The model under review builds one solid part; all positions refer to its coordinate system, in mm. A direction names the side the tool comes from. Round coordinates to 2 decimals unless told otherwise and drop trailing zeros. Write each loop counter-clockwise with the first axis right and the second up, starting at its lowest first coordinate (ties: lowest second). Pieces come first, ordered by that corner, then holes. Notation, with made-up numbers: M -2,53 L 19,53 A15 ccw 19,69 Z; hole C 75.25,56.5 d10. An arc over 180 degrees is marked long. One line per item, written item: value. Start each with the question number.
1) Take a section at D-D, the plane x = 79. Write out the cut boundary in (y, z).
2) Mouldability with a two-part tool opening along X and no side actions: class faces 3 (the face through (60.81, 6.44, 7.5)), 4 (the face through (0, 0, 7)) as +X half, -X half, draft (parallel to the pull), parting line (faces both ways), or undercut.
3) Take a section at B-B, the plane y = 5.25. Write out the cut boundary in (x, z) (3 decimals).
4) Take a section at C-C, the plane z = -51.5. Write out the cut boundary in (x, y), and give its area (3 significant figures).
5) Take a section at A-A, the plane x = 0. Write out the cut boundary in (y, z) (3 decimals).
6) Wall thickness on probe 1 along Z at (x, y) = (38, 3.5); probe 2 along X at (y, z) = (10, 66); probe 3 along X at (y, z) = (4.75, -38): over which ranges is each line inside the solid? List them lowest first.
7) For P1, Ø6, axis at x = 19.5, y = 9.5, coming from the -Z side; P2, Ø2, axis at y = 4.5, z = -45.5, coming from the +X side; P3, Ø1.5, axis at x = 16, y = 4, coming from the +Z side, all flat-tipped, find the tip position at first contact; note any pin that passes through.
8) Tool access review of faces 1 (the face through (0, 12.7, 7)), 2 (the face through (36.3, 6.4, -48.2)): name each direction out of +Z, -Z, +X, -X, +Y, -Y from which nothing blocks a thin tool from reaching the whole face with its end or side.
from build123d import *

# Parameters (mm, degrees)
SKETCH1_R           = 98.425
BOSS_EXTRUDE1_DEPTH = 12.7
CUT_EXTRUDE1_DEPTH  = 13.7


with BuildPart() as part:
    # Sketch1 → Boss-Extrude1 (new body)
    with BuildSketch(Plane(origin=(0, 0, 0), x_dir=(1, 0, 0), z_dir=(0, 1, 0))):
        Circle(SKETCH1_R)
    extrude(amount=BOSS_EXTRUDE1_DEPTH)

    # Sketch2 → Cut-Extrude1 (cut, through all)
    with BuildSketch(Plane(origin=(0, 12.7, 0), x_dir=(1, 0, 0), z_dir=(0, 1, 0))):
        with BuildLine():
            Line((21.383254088, 20.544146731), (61.581662722, 68.450744637))
            ThreePointArc((61.581662722, 68.450744637), (86.522198059, 31.491504697), (91.173581053, -12.852382775))
            Line((91.173581053, -12.852382775), (29.586045941, -1.992838659))
            ThreePointArc((29.586045941, -1.992838659), (27.864786272, 10.141952787), (21.383254088, 20.544146731))
        make_face()
        with BuildLine():
            Line((16.518871875, 24.625848052), (56.717280509, 72.532445958))
            ThreePointArc((56.717280509, 72.532445958), (15.988655959, 90.676173859), (-28.489252402, 87.556656643))
            Line((-28.489252402, 87.556656643), (-7.100125924, 28.790514622))
            ThreePointArc((-7.100125924, 28.790514622), (5.149204378, 29.202589176), (16.518871875, 24.625848052))
        make_face()
        with BuildLine():
            Line((-13.067174066, 26.618686712), (-34.456300544, 85.384828733))
            ThreePointArc((-34.456300544, 85.384828733), (-70.5335421, 59.184669162), (-90.070915125, 19.105912006))
            Line((-90.070915125, 19.105912006), (-28.483380012, 8.246367891))
            ThreePointArc((-28.483380012, 8.246367891), (-22.715581894, 19.060636389), (-13.067174066, 26.618686712))
        make_face()
        with BuildLine():
            Line((-29.586045941, 1.992838659), (-91.173581053, 12.852382775))
            ThreePointArc((-91.173581053, 12.852382775), (-86.522198059, -31.491504697), (-61.581662722, -68.450744637))
            Line((-61.581662722, -68.450744637), (-21.383254088, -20.544146731))
            ThreePointArc((-21.383254088, -20.544146731), (-27.864786272, -10.141952787), (-29.586045941, 1.992838659))
        make_face()
        with BuildLine():
            Line((-16.518871875, -24.625848052), (-56.717280509, -72.532445958))
            ThreePointArc((-56.717280509, -72.532445958), (-15.988655959, -90.676173859), (28.489252402, -87.556656643))
            Line((28.489252402, -87.556656643), (7.100125924, -28.790514622))
            ThreePointArc((7.100125924, -28.790514622), (-5.149204378, -29.202589176), (-16.518871875, -24.625848052))
        make_face()
        with BuildLine():
            Line((13.067174066, -26.618686712), (34.456300544, -85.384828733))
            ThreePointArc((34.456300544, -85.384828733), (70.5335421, -59.184669162), (90.070915125, -19.105912006))
            Line((90.070915125, -19.105912006), (28.483380012, -8.246367891))
            ThreePointArc((28.483380012, -8.246367891), (22.715581894, -19.060636389), (13.067174066, -26.618686712))
        make_face()
    extrude(amount=-CUT_EXTRUDE1_DEPTH, mode=Mode.SUBTRACT)


solid = part.part
Checked values:
1. outline: M 0,-58.71 L 12.7,-58.71 L 12.7,-47.29 L 0,-47.29 Z; M 0,10.71 L 12.7,10.71 L 12.7,17.15 L 0,17.15 Z; M 0,47.29 L 12.7,47.29 L 12.7,58.71 L 0,58.71 Z
2. face 3: undercut
2. face 4: draft
3. outline: C 0,0 d196.85; hole M -91.174,-12.852 L -29.586,-1.993 A29.653 cw -21.383,20.544 L -61.582,68.451 A92.075 ccw Z; hole M -90.071,-19.106 A92.075 ccw -34.456,-85.385 L -13.067,-26.619 A29.653 cw -28.483,-8.246 Z; hole M -56.717,72.532 L -16.519,24.626 A29.653 cw 7.1,28.791 L 28.489,87.557 A92.075 ccw Z; hole M -28.489,-87.557 A92.075 ccw 56.717,-72.532 L 16.519,-24.626 A29.653 cw -7.1,-28.791 Z; hole M 13.067,26.619 A29.653 cw 28.483,8.246 L 90.071,19.106 A92.075 ccw 34.456,85.385 Z; hole M 21.383,-20.544 L 61.582,-68.451 A92.075 ccw 91.174,12.852 L 29.586,1.993 A29.653 cw Z
4. outline: M -83.88,0 L -76.33,0 L -76.33,12.7 L -83.88,12.7 Z; M -22.12,0 L -15.37,0 L -15.37,12.7 L -22.12,12.7 Z; M 39.07,0 L 47.36,0 L 47.36,12.7 L 39.07,12.7 Z; M 76.33,0 L 83.88,0 L 83.88,12.7 L 76.33,12.7 Z
4. area: 383 mm2
5. outline: M 0,-98.425 L 12.7,-98.425 L 12.7,-92.075 L 0,-92.075 Z; M 0,-29.653 L 12.7,-29.653 L 12.7,29.653 L 0,29.653 Z; M 0,92.075 L 12.7,92.075 L 12.7,98.425 L 0,98.425 Z
6. probe 1: z = -90.79 to -83.87, -50.23 to -40.35, 3.48 to 9.92, 83.87 to 90.79
6. probe 2: x = -73.02 to -64.2, -59.53 to -51.24, 20.64 to 27.4, 64.2 to 73.02
6. probe 3: x = -90.79 to -83.87, -17.21 to -10.45, 27.74 to 36.03, 83.87 to 90.79
7. P1: stops at z = -97.03
7. P2: stops at x = 87.79
7. P3: stops at z = 97.24
8. face 1: +Z, -Z, +X, -X, +Y
8. face 2: +Y, -Y
